Geometry: final body of the model. Coordinates: model frame, mm. A direction names the side the tool comes from. Coordinates: 2 decimals unless noted, no trailing zeros. Loops run counter-clockwise (first coordinate to the right, second up) from the corner with the lowest first, then second, coordinate; pieces in that order, holes last. Notation, with made-up numbers: (-37.75, -22) -> (-30.75, -22) arc R25 cw to (-30.75, 6) -> close; hole circle Ø2 at (2.25, -33). An arc over 180 degrees is marked (long way). One line per item, written item: value. Start each with the question number.
Item 1: Section query A-A on y = 34. Return loops of the section in (x, z), then the cut area to 3 significant figures.
Item 2: Section query C-C on z = 33. Return loops of the section in (x, y).
Item 3: Section query B-B on y = -25. Return loops of the section in (x, z), then the cut area to 3 significant figures.
Item 4: Section query D-D on z = 6. Return loops of the section in (x, y), then the cut area to 3 significant figures.
Item 5: Contact query for flat-ended pins moving along their axis: pin 1 Ø0.8 at (x, y) = (-5.5, -30.5) entering from +Z; pin 2 Ø4 at (x, y) = (43.5, 26) entering from +Z; pin 3 Ø0.5 at (y, z) = (-30.5, 12) entering from -X. Output: stop coordinate, or through.
Item 6: Set-up query: faces 1 (the flat face through (-1, -9, 36)), 2 (the flat face through (14.27, 4, 26)), 3 (the flat face through (-16, 13, 18)). Return all of +Z, -Z, +X, -X, +Y, -Y with unobstructed straight access to the full face (end or side cutting, diameter ignored); none if empty.
Item 7: Ray query, probe 1 along X at (y, z) = (-11.5, 5); probe 2 along X at (y, z) = (16.5, 8); probe 3 along Z at (x, y) = (0, 34.5). Return the intervals inside material, ascending. Write a range as from..to.
Item 8: Mould query, pull axis Z, two halves, no side actions, for faces 4 (the flat face through (15, 21, 0)), 5 (the flat face through (7, -31.016, 15)), 6 (the flat face through (-1, -18, 18)). Classes: +Z half, -Z half, draft (parallel to the pull), parting line (faces both ways), or undercut.
from build123d import *

# Parameters (mm, degrees)
F0_W      = 30
F0_H      = 60
F0_W_2    = 25
F0_H_2    = 55
F1_DEPTH  = 20
F2_W      = 40
F2_H      = 15
F3_DEPTH  = 30
F5_W      = 60
F5_H      = 2
F6_DEPTH  = 10
F8_DEPTH  = 18
F10_DEPTH = 25
F12_DEPTH = 10
F13_W     = 25
F13_H     = 2
F14_DEPTH = 20
F15_W     = 25
F15_H     = 2
F16_DEPTH = 40
F18_DEPTH = 40
F4_W      = 12.4563146383
F4_H      = 17.6308546215
F19_DEPTH = 1
F20_W     = 25
F20_H     = 2.5
F21_DEPTH = 0.5
F22_W     = 2
F22_H     = 2
F23_DEPTH = 22
F26_W     = 2.5
F26_H     = 2
F27_DEPTH = 25


# Not quite as in the source:
# - the program builds the solid bodies; features that only make, move or delete a surface that nothing else refers to are left out


with BuildPart() as f1:
    # F0 (on Top) → F1 (new body)
    with BuildSketch(Plane.XY):
        with Locations((-0.72979182, -0.0160729922)):
            Rectangle(F0_W, F0_H)
        with Locations((-0.72979182, -0.0160729922)):
            Rectangle(F0_W_2, F0_H_2, mode=Mode.SUBTRACT)
    extrude(amount=F1_DEPTH)

    # F2 (on face) → F3 (join)
    with BuildSketch(Plane(origin=(-15.72979182, 0, 0), x_dir=(0, -1, 0), z_dir=(-1, 0, 0))):
        with Locations((-9.9839270078, 7.5)):
            Rectangle(F2_W, F2_H)
    extrude(amount=F3_DEPTH)

    # F5 (on face) → F6 (join)
    with BuildSketch(Plane(origin=(-15.72979182, 0, 0), x_dir=(0, -1, 0), z_dir=(-1, 0, 0))):
        with Locations((0.0160729922, 19)):
            Rectangle(F5_W, F5_H)
    extrude(amount=F6_DEPTH)

    # F7 (on face) → F8 (join)
    with BuildSketch(Plane.XY.offset(20)):
        Polygon((14.27020818, -10.0160729922), (14.27020818, 29.9839270078), (-15.72979182, 29.9839270078), (-15.72979182, -10.0160729922), (-13.22979182, -10.0160729922), (-13.22979182, 27.4839270078), (11.77020818, 27.4839270078), (11.77020818, -10.0160729922), align=None)
    extrude(amount=F8_DEPTH)

    # F9 (on face) → F10 (join)
    with BuildSketch(Plane(origin=(0, 29.9839270078, 0), x_dir=(-1, 0, 0), z_dir=(0, 1, 0))):
        Polygon((45.72979182, 0), (45.72979182, 15), (15.72979182, 15), (-14.27020818, 15), (-14.27020818, 0), align=None)
    extrude(amount=F10_DEPTH)

    # F11 (on face) → F12 (join)
    with BuildSketch(Plane(origin=(0, 29.9839270078, 0), x_dir=(-1, 0, 0), z_dir=(0, 1, 0))):
        Polygon((25.72979182, 18), (25.72979182, 20), (15.72979182, 20), (-14.27020818, 20), (-14.27020818, 18), (15.72979182, 18), align=None)
    extrude(amount=F12_DEPTH)

    # F13 (on face) → F14 (join)
    with BuildSketch(Plane(origin=(0, -27.5160729922, 0), x_dir=(-1, 0, 0), z_dir=(0, 1, 0))):
        with Locations((0.72979182, 19)):
            Rectangle(F13_W, F13_H)
    extrude(amount=F14_DEPTH)

    # F15 (on face) → F16 (join)
    with BuildSketch(Plane.XZ.offset(-27.4839270078)):
        with Locations((-0.72979182, 12)):
            Rectangle(F15_W, F15_H)
    extrude(amount=F16_DEPTH)

    # F17 (on face) → F18 (join)
    with BuildSketch(Plane.YZ.offset(14.27020818)):
        Polygon((54.7944166925, 15), (29.9839270078, 15), (-30.0160729922, 15), (-30.0160729922, 0), (54.9839270078, 0), align=None)
    extrude(amount=F18_DEPTH)

    # F4 (on face) → F19 (join)
    with BuildSketch(Plane.XZ.offset(30.0160729922)):
        with Locations((-6.2281573191, 8.8154273108)):
            Rectangle(F4_W, F4_H)
        Polygon((12.1112056077, 11.4192906767), (12.1112056077, 17.6308546215), (2.0312797278, 17.6308546215), (2.0312797278, 11.5545932204), align=None)
    extrude(amount=F19_DEPTH)

    # F20 (on face) → F21 (join)
    with BuildSketch(Plane.XY.offset(20)):
        with Locations((-0.72979182, -8.7660729922)):
            Rectangle(F20_W, F20_H)
    extrude(amount=F21_DEPTH)

    # F22 (on face) → F23 (join)
    with BuildSketch(Plane.XZ.offset(10.0160729922)):
        with Locations((13.27020818, 37)):
            Rectangle(F22_W, F22_H)
        with Locations((-14.72979182, 37)):
            Rectangle(F22_W, F22_H)
    extrude(amount=F23_DEPTH)

    # F26 (on face) → F27 (join)
    with BuildSketch(Plane(origin=(11.77020818, 0, 0), x_dir=(0, -1, 0), z_dir=(-1, 0, 0))):
        with Locations((8.7660729922, 37)):
            Rectangle(F26_W, F26_H)
    extrude(amount=F27_DEPTH)


solid = f1.part
Reply:
1. outline: (-45.73, 0) -> (54.27, 0) -> (54.27, 15) -> (-45.73, 15) -> close; (-25.73, 18) -> (14.27, 18) -> (14.27, 20) -> (-25.73, 20) -> close
1. area: 1,580 mm²
2. outline: (-15.73, -10.02) -> (-13.23, -10.02) -> (-13.23, 27.48) -> (11.77, 27.48) -> (11.77, -10.02) -> (14.27, -10.02) -> (14.27, 29.98) -> (-15.73, 29.98) -> close
3. outline: (-25.73, 18) -> (-15.73, 18) -> (-15.73, 0) -> (-13.23, 0) -> (-13.23, 18) -> (11.77, 18) -> (11.77, 0) -> (54.27, 0) -> (54.27, 15) -> (14.27, 15) -> (14.27, 20) -> (-25.73, 20) -> close; (-15.73, 36) -> (-13.73, 36) -> (-13.73, 38) -> (-15.73, 38) -> close; (12.27, 36) -> (14.27, 36) -> (14.27, 38) -> (12.27, 38) -> close
3. area: 778 mm²
4. outline: (-45.73, -10.02) -> (-15.73, -10.02) -> (-15.73, -30.02) -> (-12.46, -30.02) -> (-12.46, -31.02) -> (0, -31.02) -> (0, -30.02) -> (54.27, -30.02) -> (54.27, 54.91) -> (14.27, 54.91) -> (14.27, 54.98) -> (-45.73, 54.98) -> close; hole (-13.23, -27.52) -> (11.77, -27.52) -> (11.77, 27.48) -> (-13.23, 27.48) -> close
4. area: 6,530 mm²
5. pin 1: stops at z = 17.63
5. pin 2: stops at z = 15
5. pin 3: stops at x = -12.46
6. face 1: -Y
6. face 2: +Z, +X, +Y, -Y
6. face 3: -X, +Y
7. probe 1: x = -15.73..-13.23, 11.77..54.27
7. probe 2: x = -45.73..-13.23, 11.77..54.27
7. probe 3: z = 0..15, 18..20
8. face 4: -Z half
8. face 5: draft
8. face 6: undercut
